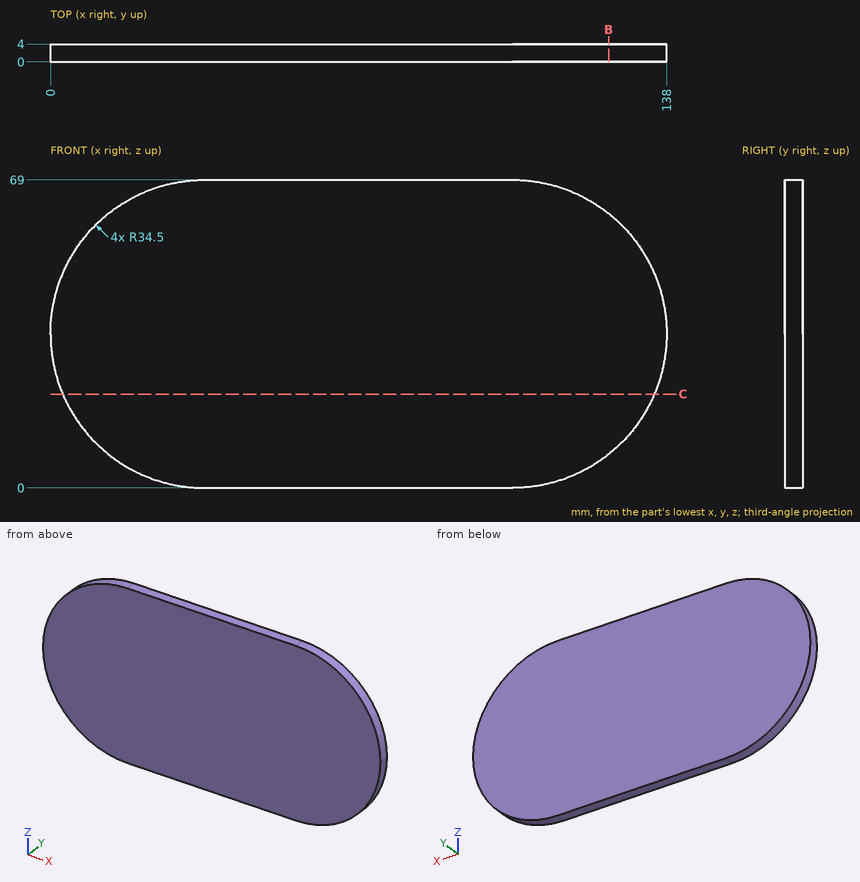
Design review of the part shown in the three views and the two pictorial views. Dimensions are in mm from the part's minimum x, y and z. Round coordinates to 2 decimals unless told otherwise and drop trailing zeros. Order: outer loops, then holes, each group sorted by start corner. A loop starts at its lowest first (then second) coordinate and runs counter-clockwise, first axis right, second up. Notation, with made-up numbers: (5.5, 15.25) - (53.5, 15.25) arc R13 ccw to (53.5, 37.25) - close; hole circle Ø9 at (38, 6). An arc over 180 degrees is marked (long way). Answer in a Markdown table with one row per item.
(1) Take a section at B-B on x = 125. Write out the cut boundary in (y, z), plus the area to 3 significant figures.
Result set:
| item | result |
|---|---|
| outline | (0, 7.52) - (4, 7.52) - (4, 61.48) - (0, 61.48) - close |
| area | 216 mm2 |
(2) For line 1 (X direction, y = 0.6, z = 50.5); line 2 (X direction, y = 1.2, z = 25.5); line 3 (Z direction, x = 26, y = 0.9), list the stretches that pass through material, from the lowest coordinate up. Write a range as from..to.
Result set:
| item | result |
|---|---|
| line 1 | x = 3.93..134.07 |
| line 2 | x = 1.19..136.81 |
| line 3 | z = 1.06..67.94 |
(3) Clearance check with flat-ended pins moving along their axes: P1, Ø3, axis at x = 90.5, z = 8.5, coming from the -Y side; P2, Ø1.5, axis at y = 2.5, z = 49.5, coming from the -X side; P3, Ø1.5, axis at y = 1, z = 51.5, coming from the -X side. State where each tip first meets the part, or that it passes through.
Result set:
| item | result |
|---|---|
| P1 | stops at y = 0 |
| P2 | stops at x = 3.08 |
| P3 | stops at x = 4.07 |
(4) Take a section at C-C on z = 21. Write out the cut boundary in (x, y), plus the area to 3 significant figures.
Result set:
| item | result |
|---|---|
| outline | (2.75, 0) - (135.25, 0) - (135.25, 4) - (2.75, 4) - close |
| area | 530 mm2 |
